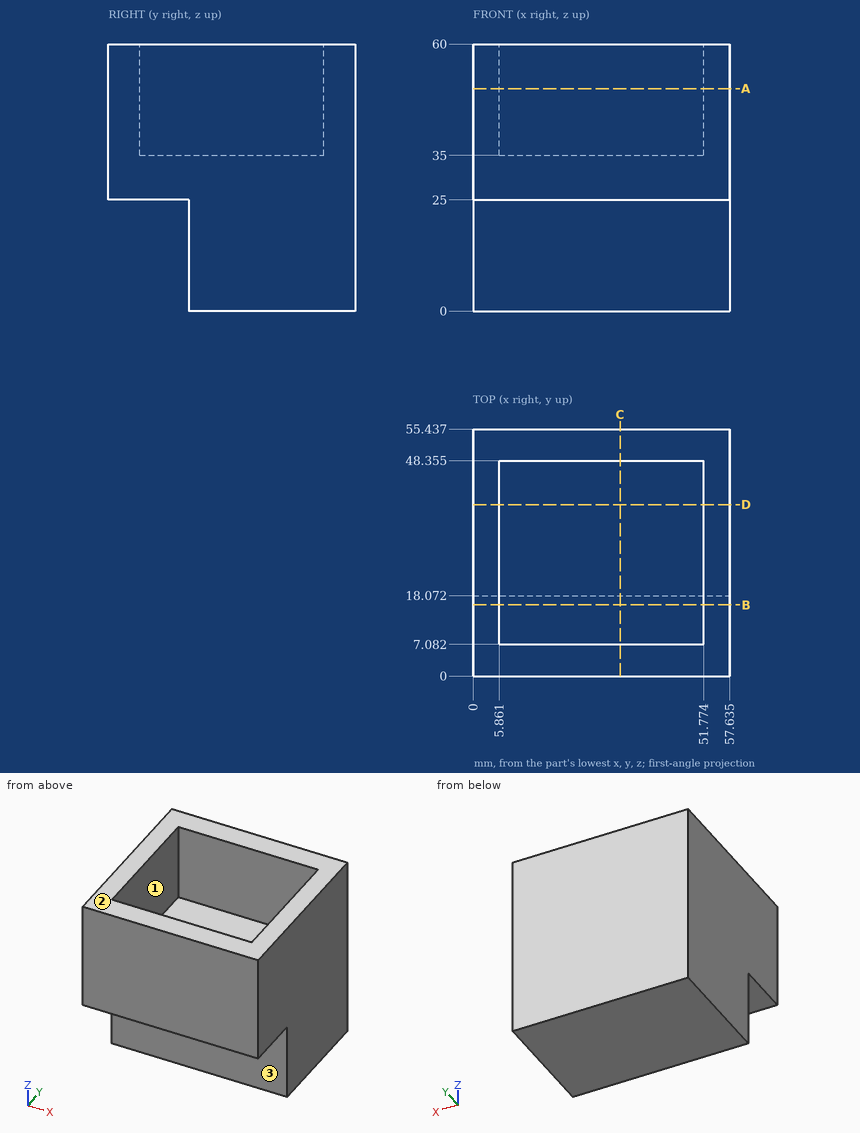
Job drawing, mm, ordinate dimensions from the low corner. One solid piece. A direction names the side the tool comes from. Coordinates: 2 decimals unless noted, no trailing zeros. Write each loop counter-clockwise with the first axis right and the second up, starting at its lowest first coordinate (ties: lowest second). Pieces come first, ordered by that corner, then holes.
Item 1: Slice it at D-D (y = 38.5). Write the cut outline in (x, z) (1 decimal).
Item 2: Pin check, flat tips, straight feed: pin 1 (5.5 mm diameter, centred on x = 24.5, y = 10.5, fed in from -Z); pin 2 (8 mm diameter, centred on x = 14, y = 13.5, fed in from +Z); pin 3 (4 mm diameter, centred on y = 16, z = 19.5, fed in from +X) (3 decimals); pin 4 (7.5 mm diameter, centred on x = 29, z = 9, fed in from -Y). Stop position of each tip, or through.
Item 3: Slice it at B-B (y = 16). Write the cut outline in (x, z) (1 decimal).
Item 4: Probe line 1 (Y direction, x = 33, z = 53) (1 decimal); line 2 (X direction, y = 34, z = 47.5) (1 decimal); line 3 (Z direction, x = 2, y = 6). List the from-to ranges inside material, lowest first.
Item 5: Which spindle directions (+Z, -Z, +X, -X, +Y, -Y) get a long thin tool onto all of the face, cutting with end or side? Do the marked faces 1, 2 and 3. Say none if no direction does.
Item 6: Slice it at C-C (x = 33). Write the cut outline in (y, z) (1 decimal).
Item 7: Slice it at A-A (z = 50). Write the cut outline in (x, y) (1 decimal).
Results found:
1. outline: (0, 0) - (57.6, 0) - (57.6, 60) - (51.8, 60) - (51.8, 35) - (5.9, 35) - (5.9, 60) - (0, 60) - close
2. pin 1: stops at z = 25
2. pin 2: stops at z = 35
2. pin 3: passes through
2. pin 4: stops at y = 18.07
3. outline: (0, 25) - (57.6, 25) - (57.6, 60) - (51.8, 60) - (51.8, 35) - (5.9, 35) - (5.9, 60) - (0, 60) - close
4. line 1: y = 0 to 7.1, 48.4 to 55.4
4. line 2: x = 0 to 5.9, 51.8 to 57.6
4. line 3: z = 25 to 60
5. face 1: +Z
5. face 2: +Z, +X, -X, +Y, -Y
5. face 3: -Z, +X, -X, -Y
6. outline: (0, 25) - (18.1, 25) - (18.1, 0) - (55.4, 0) - (55.4, 60) - (48.4, 60) - (48.4, 35) - (7.1, 35) - (7.1, 60) - (0, 60) - close
7. outline: (0, 0) - (57.6, 0) - (57.6, 55.4) - (0, 55.4) - close; hole (5.9, 7.1) - (51.8, 7.1) - (51.8, 48.4) - (5.9, 48.4) - close
